```python
from build123d import *

# Parameters (mm, degrees)
SKETCH_1_W          = 6
SKETCH_1_H          = 41.5
SKETCH_1_R          = 1.6
EXTRUDE_1_DEPTH     = 3
EXTRUDE_2_DEPTH     = 41.5
EXTRUDE_START       = 17
EXTRUDE_3_DEPTH     = 17
EXTRUDE_START_2     = 10
EXTRUDE_4_DEPTH     = 10
SKETCH_6_W          = 18.75
SKETCH_6_H          = 95.5
SKETCH_6_R          = 1.6
EXTRUDE_5_DEPTH     = 3
EXTRUDE_START_3     = 75.5
EXTRUDE_6_DEPTH     = 75.5
SKETCH_8_W          = 6
SKETCH_8_H          = 41.5
CUT_EXTRUDE_1_DEPTH = 53.193150892
SKETCH_9_R          = 3.5
CUT_EXTRUDE_2_DEPTH = 3.5
FILLET_1_R          = 2
EXTRUDE_START_4     = 14
EXTRUDE_7_DEPTH     = 14
EXTRUDE_8_DEPTH     = 14
SKETCH_12_W         = 5
SKETCH_12_H         = 10
CUT_EXTRUDE_3_DEPTH = 68.942530862


with BuildPart() as part:
    # 草图1 → 凸台-拉伸1 (new body)
    with BuildSketch(Plane(origin=(0, 0, 0), x_dir=(1, 0, 0), z_dir=(0, 1, 0))):
        Rectangle(SKETCH_1_W, SKETCH_1_H)
        with Locations(Location((0, 13, 0), (0, 0, 270))):
            Circle(SKETCH_1_R, mode=Mode.SUBTRACT)
        with Locations(Location((0, -13, 0), (0, 0, 270))):
            Circle(SKETCH_1_R, mode=Mode.SUBTRACT)
    extrude(amount=EXTRUDE_1_DEPTH)

    # 草图2 → 凸台-拉伸2 (add)
    with BuildSketch(Plane.XY.offset(20.75)):
        with BuildLine():
            ThreePointArc((-5.5, -8), (-8.502155493, -0.752155493), (-15.75, 2.25))
            Line((-15.75, 2.25), (-15.75, 3))
            Line((-15.75, 3), (-5.5, 3))
            Line((-5.5, 3), (-5.5, -8))
        make_face()
        Polygon((-5.5, 3), (-5.5, -8), (-3, -8), (-3, 0), (-3, 3), align=None)
    extrude(amount=-EXTRUDE_2_DEPTH)

    # 草图4 → 凸台-拉伸3 (add)
    with BuildSketch(Plane.XY.offset(20.75).offset(EXTRUDE_START)):
        with BuildLine():
            Line((3, -8), (3, 3))
            Line((3, 3), (-15.75, 3))
            Line((-15.75, 3), (-15.75, 2.25))
            ThreePointArc((-15.75, 2.25), (-8.502155493, -0.752155493), (-5.5, -8))
            Line((-5.5, -8), (3, -8))
        make_face()
    extrude_3 = extrude(amount=-EXTRUDE_3_DEPTH)

    # 草图5 → 凸台-拉伸4 (add)
    with BuildSketch(Plane.XY.offset(37.75).offset(EXTRUDE_START_2)):
        with BuildLine():
            Line((-15.75, -18.25), (-15.75, -21.25))
            Line((-15.75, -21.25), (3, -21.25))
            Line((3, -21.25), (3, 3))
            Line((3, 3), (-15.75, 3))
            Line((-15.75, 3), (-15.75, 2.25))
            ThreePointArc((-15.75, 2.25), (-5.5, -8), (-15.75, -18.25))
        make_face()
    extrude_4 = extrude(amount=-EXTRUDE_4_DEPTH)

    # 镜向1: 凸台-拉伸3, 凸台-拉伸4 across plane
    add(extrude_3.mirror(Plane.XY))
    add(extrude_4.mirror(Plane.XY))

    # 草图6 → 凸台-拉伸5 (add)
    with BuildSketch(Plane(origin=(0, 3, 0), x_dir=(1, 0, 0), z_dir=(0, 1, 0))):
        with Locations((-6.375, 0)):
            Rectangle(SKETCH_6_W, SKETCH_6_H)
        with Locations(Location((0, -13, 0), (0, 0, 270))):
            Circle(SKETCH_6_R, mode=Mode.SUBTRACT)
        with Locations(Location((0, 13, 0), (0, 0, 270))):
            Circle(SKETCH_6_R, mode=Mode.SUBTRACT)
    extrude(amount=EXTRUDE_5_DEPTH)

    # 草图7 → 凸台-拉伸6 (add)
    with BuildSketch(Plane.XY.offset(-37.75).offset(EXTRUDE_START_3)):
        with BuildLine():
            Line((3, -8), (-5.5, -8))
            ThreePointArc((-5.5, -8), (-8.502155493, -15.247844507), (-15.75, -18.25))
            Line((-15.75, -18.25), (-15.75, -21.25))
            Line((-15.75, -21.25), (3, -21.25))
            Line((3, -21.25), (3, -8))
        make_face()
    extrude(amount=-EXTRUDE_6_DEPTH)

    # 草图8 → 切除-拉伸1 (cut, through all)
    with BuildSketch(Plane(origin=(0, -8, 0), x_dir=(1, 0, 0), z_dir=(0, 1, 0))):
        Rectangle(SKETCH_8_W, SKETCH_8_H)
    extrude(amount=-CUT_EXTRUDE_1_DEPTH, mode=Mode.SUBTRACT)

    # 草图9 → 切除-拉伸2 (cut)
    with BuildSketch(Plane(origin=(0, 6, 0), x_dir=(1, 0, 0), z_dir=(0, 1, 0))):
        with Locations((0, 13)):
            Circle(SKETCH_9_R)
        with Locations((0, -13)):
            Circle(SKETCH_9_R)
    extrude(amount=-CUT_EXTRUDE_2_DEPTH, mode=Mode.SUBTRACT)

    # 圆角1
    fillet_1_edges = [part.edges().sort_by_distance(p)[0] for p in [
        (3, 4.25, -11.197224362),
        (3, 4.25, -14.802775638),
        (3, 4.25, 14.802775638),
        (3, 4.25, 11.197224362),
    ]]
    fillet(fillet_1_edges, radius=FILLET_1_R)

    # 草图10 → 凸台-拉伸7 (add)
    with BuildSketch(Plane.XY.offset(47.75).offset(EXTRUDE_START_4)):
        with BuildLine():
            Line((-15.75, -18.25), (-15.75, -21.25))
            Line((-15.75, -21.25), (3, -21.25))
            Line((3, -21.25), (3, 6))
            Line((3, 6), (-15.75, 6))
            Line((-15.75, 6), (-15.75, 2.25))
            ThreePointArc((-15.75, 2.25), (-5.5, -8), (-15.75, -18.25))
        make_face()
    extrude(amount=-EXTRUDE_7_DEPTH)

    # 草图11 → 凸台-拉伸8 (add)
    with BuildSketch(Plane(origin=(0, 0, -47.75), x_dir=(-1, 0, 0), z_dir=(0, 0, -1))):
        with BuildLine():
            Line((15.75, 2.25), (15.75, 6))
            Line((15.75, 6), (-3, 6))
            Line((-3, 6), (-3, -21.25))
            Line((-3, -21.25), (15.75, -21.25))
            Line((15.75, -21.25), (15.75, -18.25))
            ThreePointArc((15.75, -18.25), (5.5, -8), (15.75, 2.25))
        make_face()
    extrude(amount=EXTRUDE_8_DEPTH)

    # 草图12 → 切除-拉伸3 (cut, through all)
    with BuildSketch(Plane(origin=(3, 0, 0), x_dir=(0, 0, -1), z_dir=(1, 0, 0))):
        with Locations((45.99, -16.25)):
            Rectangle(SKETCH_12_W, SKETCH_12_H)
        with Locations((-45.99, -16.25)):
            Rectangle(SKETCH_12_W, SKETCH_12_H)
    extrude(amount=-CUT_EXTRUDE_3_DEPTH, mode=Mode.SUBTRACT)


solid = part.part
```
Model file for the job. Use its own axes, mm. A direction names the side the tool comes from. Coordinates: 2 decimals unless noted, no trailing zeros. Loops run counter-clockwise (first coordinate to the right, second up) from the corner with the lowest first, then second, coordinate; pieces in that order, holes last. Notation, with made-up numbers: M -1.5,-21 L 5.5,-21 A21 ccw 5.5,6 Z; hole C 52.25,12.25 d5. An arc over 180 degrees is marked long. Use CSV: the item, a comma, the result in double quotes. Start each with the question number.
1. Flat gauge pins, fed straight in: pin 1 (10.5 mm diameter, centred on y = -6.5, z = 3.5, fed in from +X); pin 2 (4 mm diameter, centred on x = 0, z = -13, fed in from +Y); pin 3 (2.5 mm diameter, centred on x = -2, z = -46.5, fed in from -Y); pin 4 (3 mm diameter, centred on x = -13, y = -14.5, fed in from +Z). Where does each tip first touch, or does it go through?
2. Band-saw the part on D-D, the plane y = -2.5. List the corners of the cut face in (x, z), then the cut area to 3 significant figures.
3. Band-saw the part on C-C, the plane y = -13.25. List the corners of the cut face in (x, z).
4. Probe probe 1 along Z at (x, y) = (0, 4.95); probe 2 along Z at (x, y) = (-2.25, -18.5); probe 3 along X at (y, z) = (-19.25, -5). List the from-to ranges inside material, lowest first. Write a range as [from, to].
5. Band-saw the part on A-A, the plane z = 13. List the corners of the cut face in (x, y).
6. Two-plate mould, pull along X, no slides. Class faces 1 (the cylindrical face through (-3.5, 4.3, -13.1)), 2 (the flat face through (0, -10, 20.75)), 3 (the flat face through (-15.75, -20, 1)): pulls with the +X half, pulls with the -X half, needs draft (parallel to the pull), parting line crosses it, or undercut.
7. Tool access for faces 4 (the flat face through (-15.75, -20, 55)), 5 (the cylindrical face through (-3.5, 4.3, 12.9)), 6 (the flat face through (-8, -21.25, 1)), 7 (the flat face through (0, -10, -20.75)), 8 (the flat face through (-1, -11.25, -46)): list every direction of +Z, -Z, +X, -X, +Y, -Y with a clear straight run to the whole face (end or side of a thin tool).
8. Band-saw the part on B-B, the plane x = -8. List the corners of the cut face in (y, z).
Entries:
1,pin 1,"stops at x = -3"
1,pin 2,"stops at y = 2.5"
1,pin 3,"stops at y = -11.25"
1,pin 4,"passes through"
2,outline,"M -7.1,-61.75 L 3,-61.75 L 3,-20.75 L -3,-20.75 L -3,20.75 L 3,20.75 L 3,61.75 L -7.1,61.75 Z"
2,area,"998 mm2"
3,outline,"M -6.95,-61.75 L 3,-61.75 L 3,-48.49 L -6.95,-48.49 Z; M -6.95,-43.49 L 3,-43.49 L 3,-20.75 L -3,-20.75 L -3,20.75 L 3,20.75 L 3,43.49 L -6.95,43.49 Z; M -6.95,48.49 L 3,48.49 L 3,61.75 L -6.95,61.75 Z"
4,probe 1,"z = [-61.75, -16.5], [-9.5, 9.5], [16.5, 61.75]"
4,probe 2,"z = [-61.75, -48.49], [-43.49, -20.75], [20.75, 43.49], [48.49, 61.75]"
4,probe 3,"x = [-15.75, -3]"
5,outline,"M -15.75,-21.25 L -3,-21.25 L -3,0 L -1.6,0 L -1.6,2.5 L -3.5,2.5 L -3.5,6 L -15.75,6 L -15.75,2.25 A10.25 cw -15.75,-18.25 Z; M 1.6,0 L 3,0 L 3,2.5 L 1.6,2.5 Z"
6,face 1,"undercut"
6,face 2,"needs draft"
6,face 3,"pulls with the -X half"
7,face 4,"+Z, -Z, -X, +Y, -Y"
7,face 5,"+Y"
7,face 6,"+Z, -Z, +X, -X, -Y"
7,face 7,"+X, -Y"
7,face 8,"+X, -X, -Y"
8,outline,"M -21.25,-61.75 L -14.71,-61.75 L -14.71,-48.49 L -21.25,-48.49 Z; M -21.25,-43.49 L -14.71,-43.49 L -14.71,43.49 L -21.25,43.49 Z; M -21.25,48.49 L -14.71,48.49 L -14.71,61.75 L -21.25,61.75 Z; M -1.29,-61.75 L 6,-61.75 L 6,61.75 L -1.29,61.75 Z"
